from build123d import *

# Parameters (mm, degrees)
BOSS_EXTRUDE1_DEPTH = 25
FILLET1_RADIUS      = 12.5
FILLET1_LENGTH      = 3
FILLET2_RADIUS      = 12.5
FILLET2_LENGTH      = 3
CUT_EXTRUDE1_DEPTH  = 89.639720216
CUT_EXTRUDE2_REACH  = 90.64


with BuildPart() as part:
    # Sketch1 → Boss-Extrude1 (new body)
    with BuildSketch(Plane(origin=(0, 0, 0), x_dir=(1, 0, 0), z_dir=(0, 1, 0))):
        with BuildLine():
            Line((0, 0), (0, -62))
            ThreePointArc((0, -62), (0.585786438, -63.414213562), (2, -64))
            Line((2, -64), (54, -64))
            ThreePointArc((54, -64), (55.414213562, -63.414213562), (56, -62))
            Line((56, -62), (56, 0))
            Line((56, 0), (53, 0))
            Line((53, 0), (53, -61))
            Line((53, -61), (3, -61))
            Line((3, -61), (3, 0))
            Line((3, 0), (0, 0))
        make_face()
    extrude(amount=BOSS_EXTRUDE1_DEPTH)

    # Fillet1: full round fillet: the end face becomes a half cylinder, R = half its width
    fillet1_face = Plane((1.5, 12.5, 0), x_dir=(-1, 0, 0), z_dir=(0, 0, -1))  # on the end face: x along it, z out of the body
    fillet1_slab = fillet1_face.offset(-FILLET1_RADIUS / 2) * Box(FILLET1_LENGTH, 2 * FILLET1_RADIUS, FILLET1_RADIUS, mode=Mode.PRIVATE)  # the body's end, R deep
    fillet1_round = Plane((1.5, 12.5, 12.5), x_dir=(0, 0, -1), z_dir=(-1, 0, 0)) * Cylinder(FILLET1_RADIUS, FILLET1_LENGTH, mode=Mode.PRIVATE)  # its axis R under the face
    add(fillet1_slab - fillet1_round, mode=Mode.SUBTRACT)

    # Fillet2: full round fillet: the end face becomes a half cylinder, R = half its width
    fillet2_face = Plane((54.5, 12.5, 0), x_dir=(-1, 0, 0), z_dir=(0, 0, -1))  # on the end face: x along it, z out of the body
    fillet2_slab = fillet2_face.offset(-FILLET2_RADIUS / 2) * Box(FILLET2_LENGTH, 2 * FILLET2_RADIUS, FILLET2_RADIUS, mode=Mode.PRIVATE)  # the body's end, R deep
    fillet2_round = Plane((54.5, 12.5, 12.5), x_dir=(0, 0, -1), z_dir=(-1, 0, 0)) * Cylinder(FILLET2_RADIUS, FILLET2_LENGTH, mode=Mode.PRIVATE)  # its axis R under the face
    add(fillet2_slab - fillet2_round, mode=Mode.SUBTRACT)

    # Sketch3 → Cut-Extrude1 (cut, through all)
    with BuildSketch(Plane.ZY):
        with BuildLine():
            ThreePointArc((13.5, 12.5), (13.207106781, 13.207106781), (12.5, 13.5))
            Line((12.5, 13.5), (12.5, 11.5))
            ThreePointArc((12.5, 11.5), (13.207106781, 11.792893219), (13.5, 12.5))
        make_face()
        with BuildLine():
            Line((12.5, 11.5), (12.5, 13.5))
            ThreePointArc((12.5, 13.5), (11.5, 12.5), (12.5, 11.5))
        make_face()
    extrude(amount=-CUT_EXTRUDE1_DEPTH, mode=Mode.SUBTRACT)

    # Sketch4 → Cut-Extrude2 (cut, up to next)
    with BuildSketch(Plane.XY.offset(64), mode=Mode.PRIVATE) as cut_extrude2_sk1:
        with BuildLine():
            ThreePointArc((29, 12.5), (28, 13.5), (27, 12.5))
            Line((27, 12.5), (29, 12.5))
        make_face()
    cut_extrude2_tool1 = extrude(cut_extrude2_sk1.sketch, amount=-CUT_EXTRUDE2_REACH, mode=Mode.PRIVATE) & part.part
    # Sketch4 → Cut-Extrude2 (cut, up to next)
    with BuildSketch(Plane.XY.offset(64), mode=Mode.PRIVATE) as cut_extrude2_sk2:
        with BuildLine():
            Line((29, 12.5), (27, 12.5))
            ThreePointArc((27, 12.5), (28, 11.5), (29, 12.5))
        make_face()
    cut_extrude2_tool2 = extrude(cut_extrude2_sk2.sketch, amount=-CUT_EXTRUDE2_REACH, mode=Mode.PRIVATE) & part.part
    # Sketch4 → Cut-Extrude2 (cut, up to next)
    with BuildSketch(Plane.XY.offset(64), mode=Mode.PRIVATE) as cut_extrude2_sk3:
        with BuildLine():
            ThreePointArc((29, 12.5), (28, 13.5), (27, 12.5))
            Line((27, 12.5), (29, 12.5))
        make_face()
    cut_extrude2_tool3 = extrude(cut_extrude2_sk3.sketch, amount=-CUT_EXTRUDE2_REACH, mode=Mode.PRIVATE) & part.part
    # Sketch4 → Cut-Extrude2 (cut, up to next)
    with BuildSketch(Plane.XY.offset(64), mode=Mode.PRIVATE) as cut_extrude2_sk4:
        with BuildLine():
            Line((29, 12.5), (27, 12.5))
            ThreePointArc((27, 12.5), (28, 11.5), (29, 12.5))
        make_face()
    cut_extrude2_tool4 = extrude(cut_extrude2_sk4.sketch, amount=-CUT_EXTRUDE2_REACH, mode=Mode.PRIVATE) & part.part
    add(cut_extrude2_tool1.solids().sort_by_distance((28, 12.924413, 64))[0], mode=Mode.SUBTRACT)
    add(cut_extrude2_tool2.solids().sort_by_distance((28, 12.075587, 64))[0], mode=Mode.SUBTRACT)
    add(cut_extrude2_tool3.solids().sort_by_distance((28, 12.924413, 64))[0], mode=Mode.SUBTRACT)
    add(cut_extrude2_tool4.solids().sort_by_distance((28, 12.075587, 64))[0], mode=Mode.SUBTRACT)


solid = part.part
The listing builds one solid part. Answer for the finished solid, in the listing's coordinates (mm). A direction names the side the tool comes from. Give positions to 0.01 mm unless a question says otherwise; leave off trailing zeros. Loops run counter-clockwise (first coordinate to the right, second up) from the corner with the lowest first, then second, coordinate; pieces in that order, holes last. Notation, with made-up numbers: M 36,59.5 L 77,59.5 A17 ccw 77,89.5 Z; hole C -9.75,53.5 d4. An arc over 180 degrees is marked long. Answer as CSV lines item,"result".
Item 1: The part is cut by section A-A (x = 28). Give the vertices of the cut face in (y, z), and give its area (3 significant figures).
Values follow:
outline,"M 0,61 L 11.5,61 L 11.5,64 L 0,64 Z; M 13.5,61 L 25,61 L 25,64 L 13.5,64 Z"
area,"69.0 mm^2"
Item 2: The part is cut by section B-B (z = 19). Give the vertices of the cut face in (x, y).
Values follow:
outline,"M 0,0 L 3,0 L 3,25 L 0,25 Z; M 53,0 L 56,0 L 56,25 L 53,25 Z"
Item 3: The part is cut by section C-C (y = 20). Give the vertices of the cut face in (x, z), and give its area (3 significant figures).
Values follow:
outline,"M 0,2.5 L 3,2.5 L 3,61 L 53,61 L 53,2.5 L 56,2.5 L 56,62 A2 ccw 54,64 L 2,64 A2 ccw 0,62 Z"
area,"517 mm^2"
Item 4: The mould has two halves that part along X. Classify faces 3 (the flat face through (3, 12, 31)), 4 (the flat face through (56, 12, 31)), 5 (the flat face through (0, 12, 31)): released by +X, released by -X, zero draft, split by the parting line, or undercut.
Values follow:
face 3,"undercut"
face 4,"released by +X"
face 5,"released by -X"
Item 5: Which of the six approach directions +Z, -Z, +X, -X, +Y, -Y give full straight-line access (tool end or side, diameter ignored) to faces 1 (the cylindrical face through (55.4, 12.32, 63.43)), 2 (the flat face through (28, 10, 61))?
Values follow:
face 1,"+Z, +X, +Y, -Y"
face 2,"-Z, +Y, -Y"
Item 6: Given pin 1 Ø3 at (x, y) = (28, 12.5) entering from -Z, flat-ended and moving along its own axis, determine where the tip first touches the part or whether it passes through.
Values follow:
pin 1,"stops at z = 61"
Item 7: Straight lines are drawn through the part: line 1 along Y through (x, z) = (28, 61.65); line 2 along X through (y, z) = (1, 15.5); line 3 along Z through (x, y) = (52.5, 22). For each, find the intervals that lie inside material, in ascending order. Write a range as [from, to].
Values follow:
line 1,"y = [0, 11.5], [13.5, 25]"
line 2,"x = [0, 3], [53, 56]"
line 3,"z = [61, 64]"
Item 8: The part is cut by section D-D (x = 46.5). Give the vertices of the cut face in (y, z), and give its area (3 significant figures).
Values follow:
outline,"M 0,61 L 25,61 L 25,64 L 0,64 Z"
area,"75.0 mm^2"
